from build123d import *

# Parameters (mm, degrees)
BOSS_EXTRUDE1_DEPTH = 20
BOSS_EXTRUDE2_START = -3
BOSS_EXTRUDE2_DEPTH = 3


with BuildPart() as part:
    # Sketch1 → Boss-Extrude1 (new body)
    with BuildSketch(Plane.XY):
        with BuildLine():
            Line((0, 0), (0, 97.6))
            ThreePointArc((0, 97.6), (0.702943725, 99.297056275), (2.4, 100))
            Line((2.4, 100), (5.6, 100))
            ThreePointArc((5.6, 100), (7.297056275, 99.297056275), (8, 97.6))
            Line((8, 97.6), (8, 0))
            Line((8, 0), (28, 0))
            Line((28, 0), (28, 115))
            Line((28, 115), (18, 115))
            Line((18, 115), (-10, 115))
            Line((-10, 115), (-22.4, 115))
            Line((-22.4, 115), (-22.4, 0))
            Line((-22.4, 0), (0, 0))
        make_face()
        with BuildLine():
            Line((18, 109), (18, 10))
            Line((18, 10), (20, 10))
            Line((20, 10), (20, 109))
            ThreePointArc((20, 109), (20.702943725, 110.697056275), (22.4, 111.4))
            Line((22.4, 111.4), (23.2, 111.4))
            ThreePointArc((23.2, 111.4), (24.897056275, 110.697056275), (25.6, 109))
            Line((25.6, 109), (25.6, 4.8))
            ThreePointArc((25.6, 4.8), (24.897056275, 3.102943725), (23.2, 2.4))
            Line((23.2, 2.4), (12.8, 2.4))
            ThreePointArc((12.8, 2.4), (11.102943725, 3.102943725), (10.4, 4.8))
            Line((10.4, 4.8), (10.4, 103.6))
            Line((10.4, 103.6), (-2.4, 103.6))
            Line((-2.4, 103.6), (-2.4, 4.8))
            ThreePointArc((-2.4, 4.8), (-3.102943725, 3.102943725), (-4.8, 2.4))
            Line((-4.8, 2.4), (-17.6, 2.4))
            ThreePointArc((-17.6, 2.4), (-19.297056275, 3.102943725), (-20, 4.8))
            Line((-20, 4.8), (-20, 109))
            ThreePointArc((-20, 109), (-19.297056275, 110.697056275), (-17.6, 111.4))
            Line((-17.6, 111.4), (-14.8, 111.4))
            ThreePointArc((-14.8, 111.4), (-13.102943725, 110.697056275), (-12.4, 109))
            Line((-12.4, 109), (-12.4, 12))
            Line((-12.4, 12), (-10.4, 12))
            Line((-10.4, 12), (-10.4, 109))
            ThreePointArc((-10.4, 109), (-9.697056275, 110.697056275), (-8, 111.4))
            Line((-8, 111.4), (15.6, 111.4))
            ThreePointArc((15.6, 111.4), (17.297056275, 110.697056275), (18, 109))
        make_face(mode=Mode.SUBTRACT)
    extrude(amount=BOSS_EXTRUDE1_DEPTH)

    # Sketch2 → Boss-Extrude2 (add)
    with BuildSketch(Plane.XY.offset(BOSS_EXTRUDE2_START)):
        with BuildLine():
            Line((28, 115), (-22.4, 115))
            Line((-22.4, 115), (-22.4, 0))
            Line((-22.4, 0), (0, 0))
            Line((0, 0), (0, 97.6))
            ThreePointArc((0, 97.6), (0.702943725, 99.297056275), (2.4, 100))
            Line((2.4, 100), (5.6, 100))
            ThreePointArc((5.6, 100), (7.297056275, 99.297056275), (8, 97.6))
            Line((8, 97.6), (8, 0))
            Line((8, 0), (28, 0))
            Line((28, 0), (28, 115))
        make_face()
    extrude(amount=BOSS_EXTRUDE2_DEPTH)


solid = part.part
Design review of the part built by this model. Coordinates are the model's own, in mm. A direction names the side the tool comes from. Give positions to 0.01 mm unless a question says otherwise; leave off trailing zeros. Write each loop counter-clockwise with the first axis right and the second up, starting at its lowest first coordinate (ties: lowest second). Pieces come first, ordered by that corner, then holes. Notation, with made-up numbers: M 21,7.5 L 64,7.5 A23 cw 64,18.5 Z; hole C -25.5,-9 d10. An arc over 180 degrees is marked long. Answer as a JSON object with one key per item and string values. Group by question number.
1) Tool access review of faces 1 (the face through (10.4, 54, 10)), 2 (the face through (-22.4, 58, 8)), 3 (the face through (4, 100, 8)): name each direction out of +Z, -Z, +X, -X, +Y, -Y from which nothing blocks a thin tool from reaching the whole face with its end or side.
2) Clearance check with a flat-ended pin moving along its axis: pin 1 Ø1 at (x, z) = (3.5, 8) entering from -Y. State where the tip first meets the part, or that it passes through.
3) For line 1 along X through (y, z) = (101, 2.25); line 2 along X through (y, z) = (70, 4.75); line 3 along X through (y, z) = (104, 5.5), list the stretches that pass through material, from the lowest coordinate up.
4) Mouldability with a two-part tool opening along Y and no side actions: class faces 4 (the face through (18, 0, 8)), 5 (the face through (-13.122, 110.716, 9.86)), 6 (the face through (-3, 58, -3)) as released by +Y, released by -Y, zero draft, split by the parting line, or undercut.
5) We need section A-A (y = 78.5). Give the boundary of the cut face in (x, z).
Answer key:
{
 "1": {"face 1": "+Z", "face 2": "+Z, -Z, -X, +Y, -Y", "face 3": "+Z, -Z, -Y"},
 "2": {"pin 1": "stops at y = 100"},
 "3": {"line 1": "x = -22.4 to -20, -12.4 to -10.4, -2.4 to 10.4, 18 to 20, 25.6 to 28", "line 2": "x = -22.4 to -20, -12.4 to -10.4, -2.4 to 0, 8 to 10.4, 18 to 20, 25.6 to 28", "line 3": "x = -22.4 to -20, -12.4 to -10.4, 18 to 20, 25.6 to 28"},
 "4": {"face 4": "released by -Y", "face 5": "undercut", "face 6": "zero draft"},
 "5": {"outline": "M -22.4,-3 L 0,-3 L 0,20 L -2.4,20 L -2.4,0 L -10.4,0 L -10.4,20 L -12.4,20 L -12.4,0 L -20,0 L -20,20 L -22.4,20 Z; M 8,-3 L 28,-3 L 28,20 L 25.6,20 L 25.6,0 L 20,0 L 20,20 L 18,20 L 18,0 L 10.4,0 L 10.4,20 L 8,20 Z"}
}
